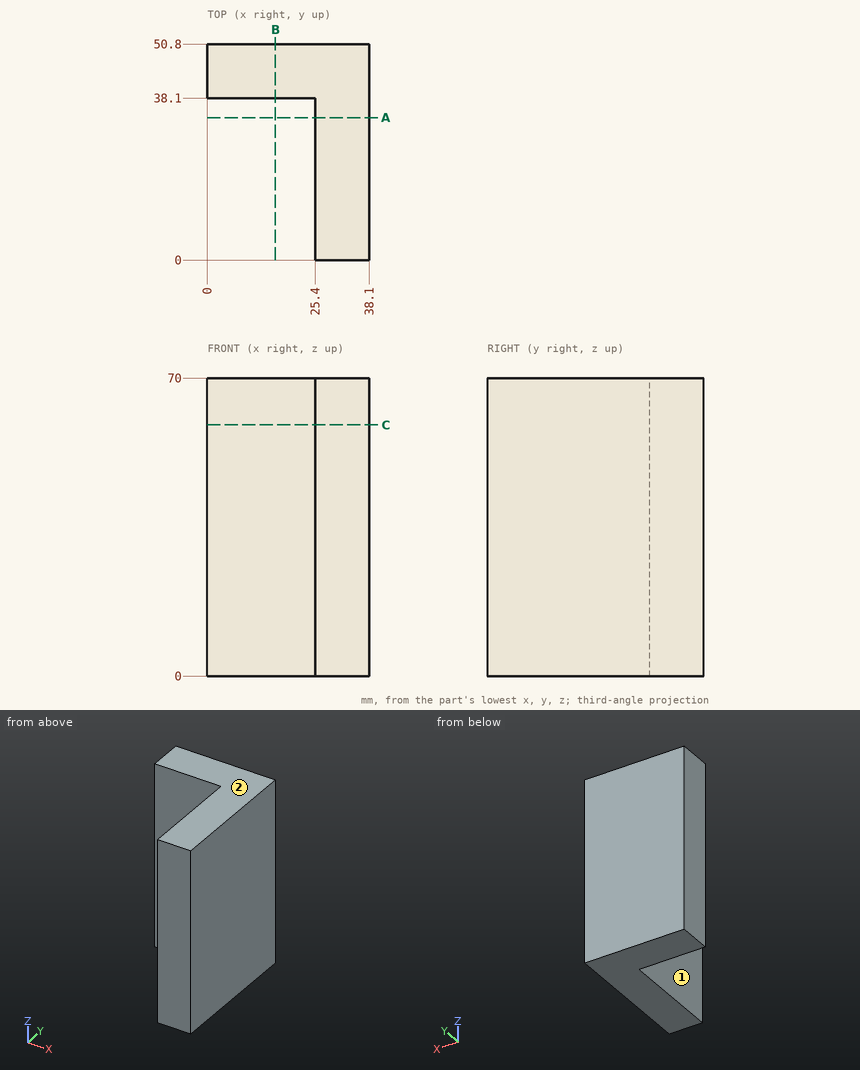
Geometry: see drawing. Coordinates: mm, zero at the bounding-box minimum. A direction names the side the tool comes from. Round coordinates to 2 decimals unless told otherwise and drop trailing zeros. Write each loop counter-clockwise with the first axis right and the second up, starting at its lowest first coordinate (ties: lowest second). Pieces come first, ordered by that corner, then holes.
Item 1: Section query A-A (y = 33.5). Return loops of the section in (x, z).
Item 2: Section query B-B (x = 16). Return loops of the section in (y, z).
Item 3: Material intervals for L1, parallel to Y at x = 22.5, z = 14.5; L2, parallel to X at y = 12.5, z = 20, sorted ascending.
Item 4: Pin query (flat end, axial travel): P1, Ø20.5, axis at x = 9.5, z = 19, coming from the -Y side; P2, Ø1.5, axis at y = 30.5, z = 22.5, coming from the -X side; P3, Ø4, axis at x = 15, y = 35, coming from the -Z side. Return the tip coordinate at first contact, or that it passes through.
Item 5: Set-up query: the marked faces 1 and 2. Return all of +Z, -Z, +X, -X, +Y, -Y with unobstructed straight access to the full face (end or side cutting, diameter ignored); none if empty.
Item 6: Section query C-C (z = 59). Return loops of the section in (x, y).
Completed:
1. outline: (25.4, 0) - (38.1, 0) - (38.1, 70) - (25.4, 70) - close
2. outline: (38.1, 0) - (50.8, 0) - (50.8, 70) - (38.1, 70) - close
3. L1: y = 38.1 to 50.8
3. L2: x = 25.4 to 38.1
4. P1: stops at y = 38.1
4. P2: stops at x = 25.4
4. P3: passes through
5. face 1: +Z, -Z, -X, -Y
5. face 2: +Z, +X, -X, +Y, -Y
6. outline: (0, 38.1) - (25.4, 38.1) - (25.4, 0) - (38.1, 0) - (38.1, 50.8) - (0, 50.8) - close
